from build123d import *

# Parameters (mm, degrees)
SKETCH1_R           = 7
BOSS_EXTRUDE1_DEPTH = 3
SKETCH2_R           = 5.9
BOSS_EXTRUDE2_DEPTH = 18
SKETCH3_W           = 0.7
SKETCH3_H           = 6
BOSS_EXTRUDE3_DEPTH = 9
SKETCH4_R           = 0.730989372
CUT_EXTRUDE1_DEPTH  = 0.7
SKETCH8_R           = 4.5
CUT_EXTRUDE2_DEPTH  = 10
SKETCH9_R           = 3
BOSS_EXTRUDE4_DEPTH = 10
SKETCH10_R          = 2
CUT_EXTRUDE3_DEPTH  = 10
FILLET3_R           = 0.7


with BuildPart() as part:
    # Sketch1 → Boss-Extrude1 (new body)
    with BuildSketch(Plane.XY):
        Circle(SKETCH1_R)
    extrude(amount=BOSS_EXTRUDE1_DEPTH)

    # Sketch2 → Boss-Extrude2 (add)
    with BuildSketch(Plane(origin=(0, 0, 0), x_dir=(-1, 0, 0), z_dir=(0, 0, -1))):
        Circle(SKETCH2_R)
    extrude(amount=BOSS_EXTRUDE2_DEPTH)

    # Sketch3 → Boss-Extrude3 (add)
    with BuildSketch(Plane(origin=(0, 0, -18), x_dir=(-1, 0, 0), z_dir=(0, 0, -1))):
        Rectangle(SKETCH3_W, SKETCH3_H)
    extrude(amount=BOSS_EXTRUDE3_DEPTH)

    # Sketch4 → Cut-Extrude1 (cut)
    with BuildSketch(Plane(origin=(0.35, 0, 0), x_dir=(0, 0, -1), z_dir=(1, 0, 0))):
        with Locations((24.802762054, 0)):
            Circle(SKETCH4_R)
    extrude(amount=-CUT_EXTRUDE1_DEPTH, mode=Mode.SUBTRACT)

    # Sketch8 → Cut-Extrude2 (cut)
    with BuildSketch(Plane.XY.offset(3)):
        Circle(SKETCH8_R)
    extrude(amount=-CUT_EXTRUDE2_DEPTH, mode=Mode.SUBTRACT)

    # Sketch9 → Boss-Extrude4 (add)
    with BuildSketch(Plane.XY.offset(-7)):
        Circle(SKETCH9_R)
    extrude(amount=BOSS_EXTRUDE4_DEPTH)

    # Sketch10 → Cut-Extrude3 (cut)
    with BuildSketch(Plane.XY.offset(3)):
        Circle(SKETCH10_R)
    extrude(amount=-CUT_EXTRUDE3_DEPTH, mode=Mode.SUBTRACT)

    # Fillet3
    fillet3_edges = [part.edges().sort_by_distance(p)[0] for p in [
        (-4.5, 0, 3),
        (-7, 0, 3),
    ]]
    fillet(fillet3_edges, radius=FILLET3_R)


solid = part.part
Read the model definition and answer for the solid it produces. Units are mm, in the model's axes. A direction names the side the tool comes from. Round coordinates to 2 decimals unless told otherwise and drop trailing zeros. Write each loop counter-clockwise with the first axis right and the second up, starting at its lowest first coordinate (ties: lowest second). Pieces come first, ordered by that corner, then holes. Notation, with made-up numbers: (-15.75, 76) - (-4.75, 76) arc R24 cw to (-4.75, 92) - close; hole circle Ø9 at (80.25, 26). An arc over 180 degrees is marked (long way). One line per question, with ' | ' between items. Start each with the question number.
1. Section D-D (z = -14.25) is taken. Determine the outline of the cut face in (x, y).
2. For a pull along X with two mould halves and no side action, classify faces 1 (the face through (6.466, -2.681, 1.134)), 2 (the face through (-2, 5, 3)), 3 (the face through (0.35, 0, -22)), 4 (the face through (-0.59, 4.46, -2.28)) as +X half, -X half, draft (parallel to the pull), parting line (faces both ways), or undercut.
3. For faces 5 (the face through (5.894, 0.259, -8.874)), 6 (the face through (0, 0.22, -25.5)), 7 (the face through (-0.35, 0, -22)), 8 (the face through (1, -2, 3)), 9 (the face through (0, 0, -7)), determine the directions among +Z, -Z, +X, -X, +Y, -Y from which every point of the face is accessible in a straight line to the end or side of a thin tool.
4. Each of these flat-tipped pins is pushed along its axis until it touches: pin 1 (3.5 mm diameter, centred on x = 0, y = 0, fed in from +Z); pin 2 (3 mm diameter, centred on y = -1, z = -21.5, fed in from +X); pin 3 (6.5 mm diameter, centred on y = -0.5, z = -20.5, fed in from -X). Where does it stop, or does it pass through?
5. Find the intervals of material crossed by probe 1 along Y at (x, z) = (0, -4.5); probe 2 along X at (y, z) = (0.5, -1.25); probe 3 along Z at (x, y) = (-2, -1), in increasing order. Write a range as [from, to].
6. Section C-C (z = -4) is taken. Determine the outline of the cut face in (x, y), and give its area (3 significant figures).
Filled in:
1) outline: circle Ø11.8 at (0, 0)
2) face 1: parting line | face 2: draft | face 3: +X half | face 4: undercut
3) face 5: -Z | face 6: +X, -X | face 7: -Z, -X, +Y, -Y | face 8: +Z, +X, -X, +Y, -Y | face 9: +Z
4) pin 1: z = -7 | pin 2: x = 0.35 | pin 3: x = -5.9
5) probe 1: [-5.9, -4.5], [-3, -2], [2, 3], [4.5, 5.9] | probe 2: [-5.88, -4.47], [-2.96, -1.94], [1.94, 2.96], [4.47, 5.88] | probe 3: [-18, 3]
6) outline: circle Ø11.8 at (0, 0); circle Ø6 at (0, 0); hole circle Ø9 at (0, 0); hole circle Ø4 at (0, 0) | area: 61.4 mm²
